The drawing under review shows one solid part. Ordinate dimensions are in mm from its lowest x, y, z. A direction names the side the tool comes from. Round coordinates to 2 decimals unless told otherwise and drop trailing zeros. Order: outer loops, then holes, each group sorted by start corner. A loop starts at its lowest first (then second) coordinate and runs counter-clockwise, first axis right, second up. Notation, with made-up numbers: M 87,-17.5 L 139,-17.5 A13 ccw 139,1.5 Z; hole C 46.25,7.5 d3. An arc over 180 degrees is marked long. Write item = value, one per line. Start each with the question number.
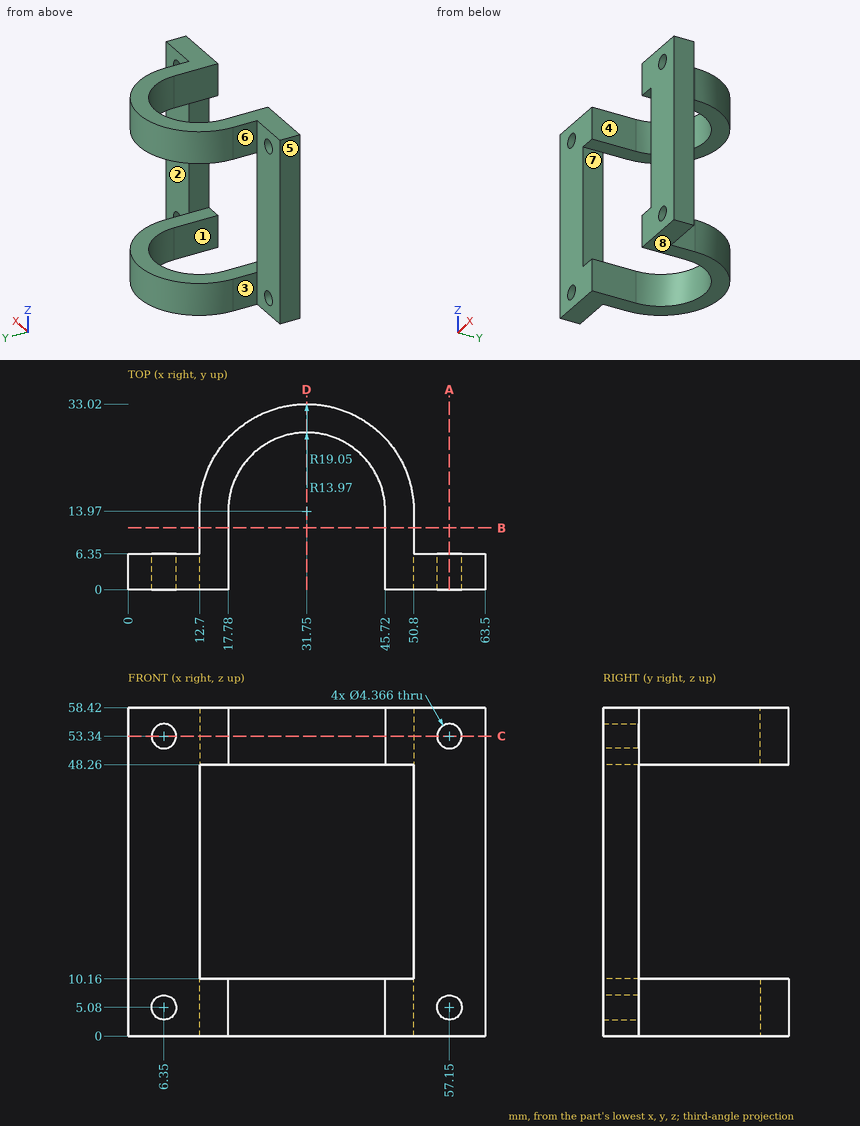
(1) For the marked faces 4, 5, 6, 7 and 8, list the 3-axis set-ups (+Z, -Z, +X, -X, +Y, -Y) from which the entire face can be reached by the end or side of a thin tool; tool diameter is ignored.
(2) Consider section B-B, the plane y = 11. Write out the cut boundary in (x, z).
(3) Insertion check: pin 1 (5 mm diameter, centred on x = 39.5, z = 8, fed in from +Y); pin 2 (4 mm diameter, centred on x = 55, z = 32, fed in from +Y); pin 3 (4 mm diameter, centred on y = 10, z = 55, fed in from -X). Each pin has a flat end and moves straight along its axis. Give the tip position at first contact, or say it passes through.
(4) Consider section C-C, the plane z = 53.34. Write out the cut boundary in (x, y).
(5) Consider section A-A, the plane x = 57.15. Write out the cut boundary in (y, z).
(6) Consider section D-D, the plane x = 31.75. Write out the cut boundary in (y, z).
(7) Draft analysis for pull direction X (two halves, no side actions). For the marked faces 1, 2 and 3, state which applies: pulls with the +X half, pulls with the -X half, needs draft (parallel to the pull), parting line crosses it, or undercut.
(8) For line 1 along Z through (x, y) = (57, 2); line 2 along X through (y, z) = (2.5, 53.34); line 3 along X through (y, z) = (6, 51.5) (1 decimal), list the stretches that pass through material, from the lowest coordinate up. Write a range as [from, to].
Completed:
q1.face_4 = +Z, -Z, -Y
q1.face_5 = +Z, -Z, -X, +Y, -Y
q1.face_6 = +Z, -Z, -X, +Y
q1.face_7 = +Y, -Y
q1.face_8 = -Z, +X, -X, +Y, -Y
q2.outline = M 12.7,0 L 17.78,0 L 17.78,10.16 L 12.7,10.16 Z; M 12.7,48.26 L 17.78,48.26 L 17.78,58.42 L 12.7,58.42 Z; M 45.72,0 L 50.8,0 L 50.8,10.16 L 45.72,10.16 Z; M 45.72,48.26 L 50.8,48.26 L 50.8,58.42 L 45.72,58.42 Z
q3.pin_1 = 32.28
q3.pin_2 = 6.35
q3.pin_3 = 12.7
q4.outline = M 0,0 L 4.17,0 L 4.17,6.35 L 0,6.35 Z; M 8.53,0 L 17.78,0 L 17.78,13.97 A13.97 cw 45.72,13.97 L 45.72,0 L 54.97,0 L 54.97,6.35 L 50.8,6.35 L 50.8,13.97 A19.05 ccw 12.7,13.97 L 12.7,6.35 L 8.53,6.35 Z; M 59.33,0 L 63.5,0 L 63.5,6.35 L 59.33,6.35 Z
q5.outline = M 0,0 L 6.35,0 L 6.35,2.9 L 0,2.9 Z; M 0,7.26 L 6.35,7.26 L 6.35,51.16 L 0,51.16 Z; M 0,55.52 L 6.35,55.52 L 6.35,58.42 L 0,58.42 Z
q6.outline = M 27.94,0 L 33.02,0 L 33.02,10.16 L 27.94,10.16 Z; M 27.94,48.26 L 33.02,48.26 L 33.02,58.42 L 27.94,58.42 Z
q7.face_1 = undercut
q7.face_2 = needs draft
q7.face_3 = pulls with the -X half
q8.line_1 = [0, 2.9], [7.26, 51.16], [55.52, 58.42]
q8.line_2 = [0, 4.17], [8.53, 17.78], [45.72, 54.97], [59.33, 63.5]
q8.line_3 = [0, 5.2], [7.5, 17.8], [45.7, 56], [58.3, 63.5]
